For this review, use the dimensioned drawing (mm, ordinates from the lowest corner) and the shaded views. A direction names the side the tool comes from. Coordinates: 2 decimals unless noted, no trailing zeros. Loops run counter-clockwise (first coordinate to the right, second up) from the corner with the lowest first, then second, coordinate; pieces in that order, holes last. Notation, with made-up numbers: (74.25, -9) - (80.25, -9) arc R35 cw to (80.25, 25) - close; hole circle Ø9 at (-38.75, -39.5). An arc over 180 degrees is marked (long way). Answer in a Markdown table with one row per item. Add a question column.
(1) For line 1 along X through (y, z) = (13, 16); line 2 along X through (y, z) = (19.5, 10.75); line 3 along Z through (x, y) = (51.5, 11), list the stretches that pass through material, from the lowest coordinate up.
(2) For P1, Ø2, axis at x = 74, y = 9, coming from the -Z side; P2, Ø1, axis at x = 62, y = 14, coming from the +Z side; P3, Ø1.5, axis at x = 84, z = 15, coming from the +Y side, all flat-tipped, find the tip position at first contact; note any pin that passes through.
(3) We need section A-A on z = 11.1. Write out the cut boundary in (x, y).
(4) We need section D-D on x = 10. Write out the cut boundary in (y, z).
(5) We need section C-C on x = 89. Write out the cut boundary in (y, z), plus the area to 3 significant figures.
(6) Machinability: for the marked faces 1 and 2, which of the approach directions +Z, -Z, +X, -X, +Y, -Y give a long, thin tool a straight path to every point of the face, cutting with its end or side? Answer none if there is none.
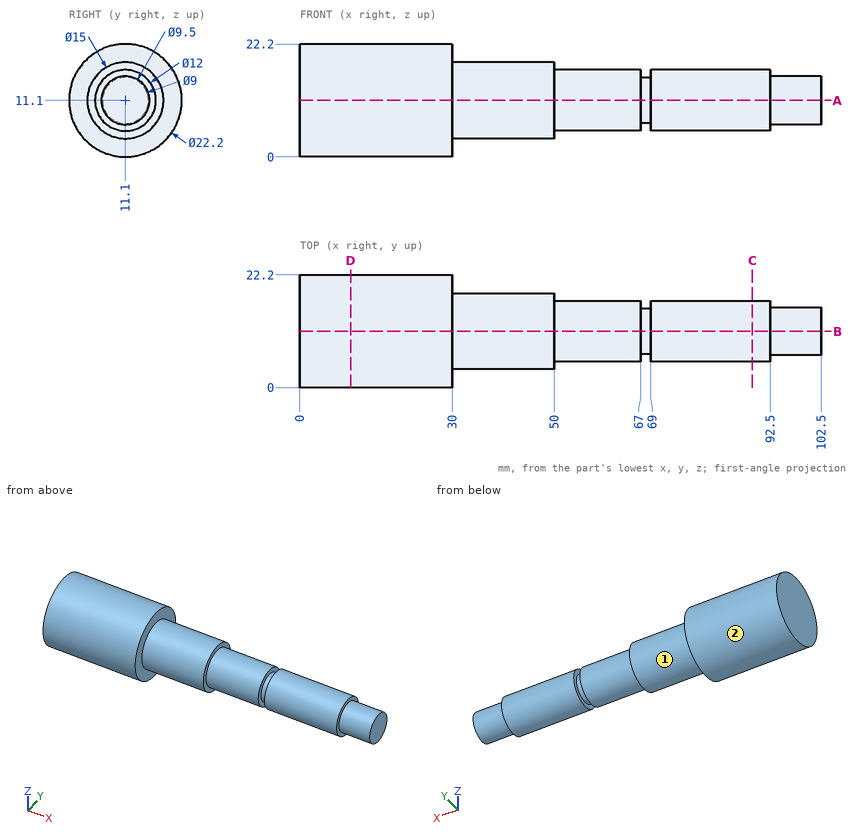
Outcome:
| question | item | result |
|---|---|---|
| 1 | line 1 | 0 to 67, 69 to 92.5 |
| 1 | line 2 | 0 to 30 |
| 1 | line 3 | 5.1 to 17.1 |
| 2 | P1 | z = 5.2 |
| 2 | P2 | z = 16.6 |
| 2 | P3 | y = 16.21 |
| 3 | outline | (0, 0) - (30, 0) - (30, 3.6) - (50, 3.6) - (50, 5.1) - (67, 5.1) - (67, 6.6) - (69, 6.6) - (69, 5.1) - (92.5, 5.1) - (92.5, 6.35) - (102.5, 6.35) - (102.5, 15.85) - (92.5, 15.85) - (92.5, 17.1) - (69, 17.1) - (69, 15.6) - (67, 15.6) - (67, 17.1) - (50, 17.1) - (50, 18.6) - (30, 18.6) - (30, 22.2) - (0, 22.2) - close |
| 4 | outline | circle Ø22.2 at (11.1, 11.1) |
| 5 | outline | circle Ø12 at (11.1, 11.1) |
| 5 | area | 113 mm² |
| 6 | face 1 | +X |
| 6 | face 2 | +X, -X |
